```python
from build123d import *

# Parameters (mm, degrees)
F0_R            = 5
F2_DEPTH        = 16
F3_R            = 6.5
F4_DEPTH        = 1
F4_COPIES_COUNT = 4
F0_R_2          = 2.5
F5_DEPTH        = 3


# Not quite as in the source:
# - a pattern or mirror of a feature is missing from the dataset's text; its kind, count and spacing are read off the source's solid


with BuildPart() as f2:
    # F0 (on Top) → F2 (new body)
    with BuildSketch(Plane.XY):
        with BuildLine():
            Line((11, -8), (11, 8))
            ThreePointArc((11, 8), (9.6176920308, 9.6176920308), (8, 11))
            Line((8, 11), (-8, 11))
            ThreePointArc((-8, 11), (-9.6176920308, 9.6176920308), (-11, 8))
            Line((-11, 8), (-11, -8))
            ThreePointArc((-11, -8), (-9.6176920308, -9.6176920308), (-8, -11))
            Line((-8, -11), (8, -11))
            ThreePointArc((8, -11), (9.6176920308, -9.6176920308), (11, -8))
        make_face()
        Circle(F0_R, mode=Mode.SUBTRACT)
    extrude(amount=F2_DEPTH)

    # F3 (on face) → F4 (cut)
    with BuildSketch(Plane.XZ.offset(11)):
        with Locations((0, 8)):
            Circle(F3_R)
    f4 = extrude(amount=-F4_DEPTH, mode=Mode.SUBTRACT)

    # F4_copies: F4 ×4 about axis
    f4_copies_axis = Axis((0, 0, 0), (0, 0, 1))
    for i in range(1, F4_COPIES_COUNT):
        add(f4.rotate(f4_copies_axis, i * 360 / F4_COPIES_COUNT), mode=Mode.SUBTRACT)

    # F0 (on Top) → F5 (join)
    with BuildSketch(Plane.XY):
        Circle(F0_R)
        Circle(F0_R_2, mode=Mode.SUBTRACT)
    extrude(amount=F5_DEPTH)


solid = f2.part
```
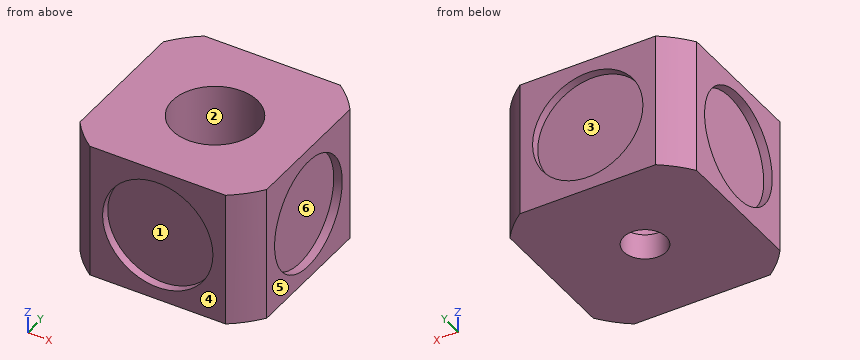
Source: CAD feature listing. Evaluate the final solid. Frame: model axes, mm. Face numbers are marked on the shaded views. A direction names the side the tool comes from. Round coordinates to 2 decimals unless told otherwise and drop trailing zeros. Loops run counter-clockwise (first coordinate to the right, second up) from the corner with the lowest first, then second, coordinate; pieces in that order, holes last. Notation, with made-up numbers: M -34,-14.5 L 25,-14.5 A32 ccw 25,17.5 Z; hole C -7.75,48 d5. An arc over 180 degrees is marked long. Use a Markdown table: item, result. Add a question column.
1. Section query C-C on z = 8. Return the cut outline in (x, y).
2. Line query: line 1 (X direction, y = 0.5, z = 14); line 2 (X direction, y = 6, z = 6.5); line 3 (Y direction, x = 1, z = 9.75). Output: solid intervals per line, ascending.
3. Mould query, pull axis Y, two halves, no side actions, for the marked faces 4, 5 and 6. Classes: pulls with the +Y half, pulls with the -Y half, needs draft (parallel to the pull), parting line crosses it, or undercut.
4. Reachability of the marked faces 1, 2 and 3 from +Z, -Z, +X, -X, +Y, -Y: full face, straight path, thin tool, end or side. Return the list, or none.
5. Section query D-D on x = 3.25. Return the cut outline in (y, z), then the cut area to 3 significant figures.
6. Contact query for flat-ended pins moving along their axis: P1, Ø9, axis at x = 0, y = 0, coming from the +Z side; P2, Ø4, axis at x = 3, z = 5, coming from the -Y side. Output: stop coordinate, or through.
7. Section query A-A on y = 0. Return the cut outline in (x, z), then the cut area to 3 significant figures.
Reported:
| question | item | result |
|---|---|---|
| 1 | outline | M -11,-8 A13.6 ccw -8,-11 L -6.5,-11 L -6.5,-10 L 6.5,-10 L 6.5,-11 L 8,-11 A13.6 ccw 11,-8 L 11,-6.5 L 10,-6.5 L 10,6.5 L 11,6.5 L 11,8 A13.6 ccw 8,11 L 6.5,11 L 6.5,10 L -6.5,10 L -6.5,11 L -8,11 A13.6 ccw -11,8 L -11,6.5 L -10,6.5 L -10,-6.5 L -11,-6.5 Z; hole C 0,0 d10 |
| 2 | line 1 | x = -10 to -4.97, 4.97 to 10 |
| 2 | line 2 | x = -10 to 10 |
| 2 | line 3 | y = -10 to -4.9, 4.9 to 10 |
| 3 | face 4 | pulls with the -Y half |
| 3 | face 5 | needs draft |
| 3 | face 6 | undercut |
| 4 | face 1 | -Y |
| 4 | face 2 | +Z |
| 4 | face 3 | +Y |
| 5 | outline | M -11,0 L 11,0 L 11,2.37 L 10,2.37 L 10,13.63 L 11,13.63 L 11,16 L 3.8,16 L 3.8,3 L -3.8,3 L -3.8,16 L -11,16 L -11,13.63 L -10,13.63 L -10,2.37 L -11,2.37 Z |
| 5 | area | 231 mm² |
| 6 | P1 | stops at z = 3 |
| 6 | P2 | stops at y = -10 |
| 7 | outline | M -11,0 L -2.5,0 L -2.5,3 L -5,3 L -5,16 L -11,16 L -11,14.5 L -10,14.5 L -10,1.5 L -11,1.5 Z; M 2.5,0 L 11,0 L 11,1.5 L 10,1.5 L 10,14.5 L 11,14.5 L 11,16 L 5,16 L 5,3 L 2.5,3 Z |
| 7 | area | 181 mm² |
